Answer from the drawing. Dimensions are ordinates in mm from the lowest x, y and z of the part. A direction names the side the tool comes from. Round coordinates to 2 decimals unless told otherwise and drop trailing zeros. Loops run counter-clockwise (first coordinate to the right, second up) from the corner with the lowest first, then second, coordinate; pieces in that order, holes last.
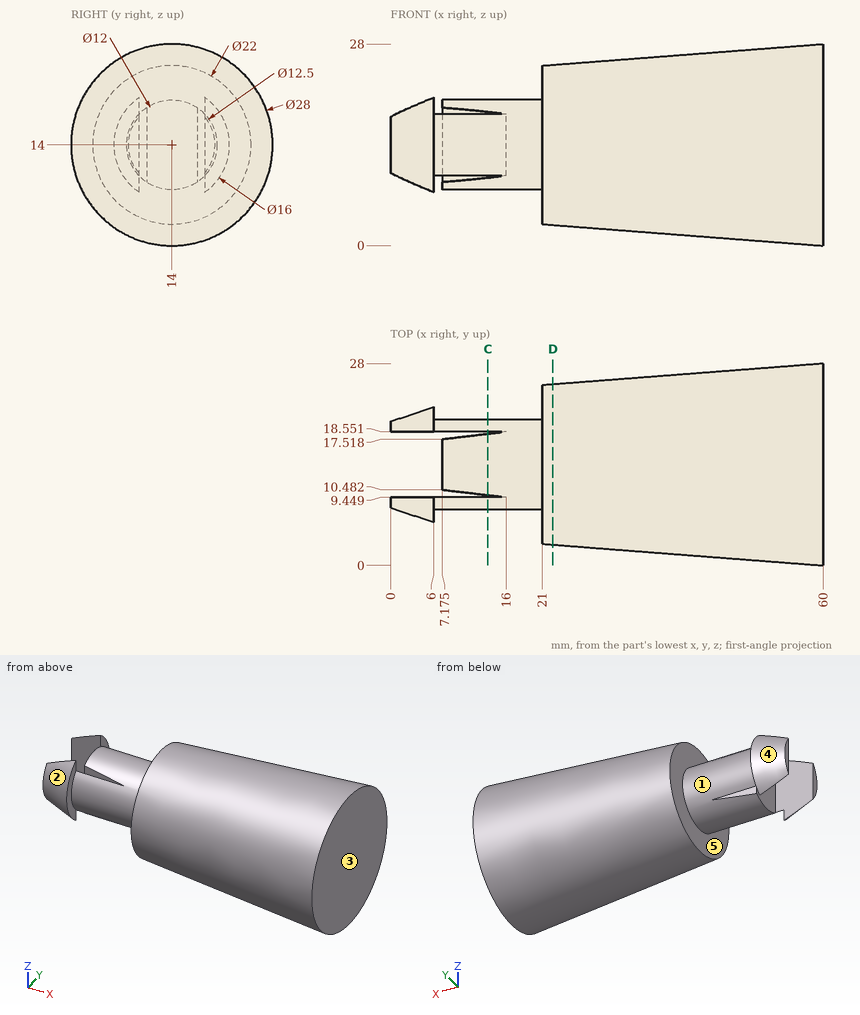
Item 1: Section C-C, the plane x = 13.5 is taken. State how many separate pieces and enclosed holes the cut face has.
Item 2: Section D-D, the plane x = 22.5 is taken. Give the vertices of the cut face in (y, z) (1 decimal).
Item 3: Determine the mould class of the marked faces 3, 4 and 5 for opening direction X: pulls with the +X half, pulls with the -X half, needs draft (parallel to the pull), parting line crosses it, or undercut.
Item 4: Each of these flat-tipped pins is pushed along its axis until it touches: P1, Ø6.5, axis at x = 4.5, z = 15.5, coming from the +Y side; P2, Ø6, axis at x = 41.5, y = 18.5, coming from the +Z side; P3, Ø5, axis at x = 20, z = 20, coming from the -Y side (1 decimal). Where does it stop, or does it pass through?
Item 5: Straight lines are drawn through the part: line 1 (X direction, y = 4, z = 13); line 2 (X direction, y = 8.5, z = 10) (1 decimal); line 3 (Y direction, x = 52.5, z = 26) (1 decimal). For each, find the intervals that lie inside material, in ascending order.
Item 6: For the marked faces 1 and 2, determine the directions among +Z, -Z, +X, -X, +Y, -Y from which every point of the face is accessible in a straight line to the end or side of a thin tool.
Answer below:
1. separate pieces: 3
1. enclosed holes: 0
2. outline: circle Ø22.2 at (14, 14)
3. face 3: pulls with the +X half
3. face 4: pulls with the -X half
3. face 5: undercut
4. P1: stops at y = 22
4. P2: stops at z = 26.55
4. P3: stops at y = 3.6
5. line 1: x = 21 to 60
5. line 2: x = 2.4 to 6, 21 to 60
5. line 3: y = 8 to 20
6. face 1: none
6. face 2: -X, -Y
